from build123d import *

# Parameters (mm, degrees)
SKETCH1_W                = 9
SKETCH1_H                = 55
SKETCH1_W_2              = 91
SKETCH1_H_2              = 5
BOSS_EXTRUDE3_DEPTH      = 5
SKETCH6_W                = 18
SKETCH6_H                = 60
BOSS_EXTRUDE4_DEPTH      = 18
SKETCH7_W                = 91
SKETCH7_H                = 5
BOSS_EXTRUDE5_DEPTH      = 100
SKETCH13_W               = 18
SKETCH13_H               = 5
CUT_EXTRUDE6_DEPTH       = 75
SKETCH16_R               = 4.2
CUT_EXTRUDE7_DEPTH       = 20
CUT_EXTRUDE8_DEPTH       = 75
CUT_EXTRUDE10_DEPTH      = 8
CUT_EXTRUDE11_DEPTH      = 22
CUT_EXTRUDE14_DEPTH      = 34
CUT_EXTRUDE14_DEPTH_BACK = 5
FILLET4_R                = 10
CUT_EXTRUDE15_DEPTH      = 24
CUT_EXTRUDE15_DEPTH_BACK = 1
SKETCH23_R               = 21
SKETCH26_R               = 1.575
CUT_EXTRUDE16_DEPTH      = 10
SKETCH27_W               = 40
SKETCH27_H               = 5
BOSS_EXTRUDE6_DEPTH      = 10


with BuildPart() as part:
    # Sketch1 → Boss-Extrude3 (new body)
    with BuildSketch(Plane.XY):
        with Locations((41, -0.737170899)):
            Rectangle(SKETCH1_W, SKETCH1_H)
        with Locations((32, -0.737170899)):
            Rectangle(SKETCH1_W, SKETCH1_H)
        with BuildLine():
            Line((27.5, 26.762829101), (0, 26.762829101))
            Line((0, 26.762829101), (0, 10.812829101))
            ThreePointArc((0, 10.812829101), (8.167083323, 7.429912424), (11.55, -0.737170899))
            ThreePointArc((11.55, -0.737170899), (8.167083323, -8.904254222), (0, -12.287170899))
            Line((0, -12.287170899), (0, -28.237170899))
            Line((0, -28.237170899), (27.5, -28.237170899))
            Line((27.5, -28.237170899), (27.5, 26.762829101))
        make_face()
        with BuildLine():
            Line((0, 10.812829101), (0, 26.762829101))
            Line((0, 26.762829101), (-27.5, 26.762829101))
            Line((-27.5, 26.762829101), (-27.5, -28.237170899))
            Line((-27.5, -28.237170899), (0, -28.237170899))
            Line((0, -28.237170899), (0, -12.287170899))
            ThreePointArc((0, -12.287170899), (-11.55, -0.737170899), (0, 10.812829101))
        make_face()
        with Locations((-32, -0.737170899)):
            Rectangle(SKETCH1_W, SKETCH1_H)
        with Locations((-41, -0.737170899)):
            Rectangle(SKETCH1_W, SKETCH1_H)
        with Locations((0, 29.262829101)):
            Rectangle(SKETCH1_W_2, SKETCH1_H_2)
    extrude(amount=BOSS_EXTRUDE3_DEPTH)

    # Sketch6 → Boss-Extrude4 (add)
    with BuildSketch(Plane(origin=(0, 0, 0), x_dir=(-1, 0, 0), z_dir=(0, 0, -1))):
        with Locations((-36.5, 1.762829101)):
            Rectangle(SKETCH6_W, SKETCH6_H)
        with Locations((36.5, 1.762829101)):
            Rectangle(SKETCH6_W, SKETCH6_H)
    extrude(amount=BOSS_EXTRUDE4_DEPTH)

    # Sketch7 → Boss-Extrude5 (add)
    with BuildSketch(Plane.XY.offset(5)):
        with Locations((0, 29.262829101)):
            Rectangle(SKETCH7_W, SKETCH7_H)
    extrude(amount=BOSS_EXTRUDE5_DEPTH)

    # Sketch13 → Cut-Extrude6 (cut)
    with BuildSketch(Plane(origin=(0, 31.762829101, 0), x_dir=(1, 0, 0), z_dir=(0, 1, 0))):
        with Locations((-36.5, 15.5)):
            Rectangle(SKETCH13_W, SKETCH13_H)
        with Locations((36.5, 15.5)):
            Rectangle(SKETCH13_W, SKETCH13_H)
    extrude(amount=-CUT_EXTRUDE6_DEPTH, mode=Mode.SUBTRACT)

    # Sketch16 → Cut-Extrude7 (cut)
    with BuildSketch(Plane(origin=(0, 31.762829101, 0), x_dir=(1, 0, 0), z_dir=(0, 1, 0))):
        with Locations(Location((-36.5, 4, 0), (0, 0, 180))):
            Circle(SKETCH16_R)
        with Locations(Location((36.5, 4, 0), (0, 0, 180))):
            Circle(SKETCH16_R)
    extrude(amount=-CUT_EXTRUDE7_DEPTH, mode=Mode.SUBTRACT)

    # Sketch17 → Cut-Extrude8 (cut)
    with BuildSketch(Plane(origin=(0, 31.762829101, 0), x_dir=(1, 0, 0), z_dir=(0, 1, 0))):
        with BuildLine():
            Line((-45.5, 13), (-45.5, 4))
            ThreePointArc((-45.5, 4), (-42.863961031, 10.363961031), (-36.5, 13))
            Line((-36.5, 13), (-45.5, 13))
        make_face()
        with BuildLine():
            ThreePointArc((-36.5, 13), (-30.136038969, 10.363961031), (-27.5, 4))
            Line((-27.5, 4), (-27.5, 13))
            Line((-27.5, 13), (-36.5, 13))
        make_face()
        with BuildLine():
            Line((27.5, 13), (27.5, 4))
            ThreePointArc((27.5, 4), (30.136038969, 10.363961031), (36.5, 13))
            Line((36.5, 13), (27.5, 13))
        make_face()
        with BuildLine():
            Line((45.5, 13), (36.5, 13))
            ThreePointArc((36.5, 13), (42.863961031, 10.363961031), (45.5, 4))
            Line((45.5, 4), (45.5, 13))
        make_face()
    extrude(amount=-CUT_EXTRUDE8_DEPTH, mode=Mode.SUBTRACT)

    # Sketch18 → Cut-Extrude10 (cut)
    with BuildSketch(Plane(origin=(0, 31.762829101, 0), x_dir=(1, 0, 0), z_dir=(0, 1, 0))):
        with BuildLine():
            ThreePointArc((-45.5, -105), (-26.743051045, -83.063543967), (-20, -55))
            Line((-20, -55), (-45.5, -55))
            Line((-45.5, -55), (-45.5, -105))
        make_face()
        with BuildLine():
            Line((-45.5, -55), (-20, -55))
            ThreePointArc((-20, -55), (-26.743051045, -26.936456033), (-45.5, -5))
            Line((-45.5, -5), (-45.5, -55))
        make_face()
        with BuildLine():
            ThreePointArc((-45.5, -105), (-26.743051045, -83.063543967), (-20, -55))
            Line((-20, -55), (-45.5, -55))
            Line((-45.5, -55), (-45.5, -105))
        make_face()
        with BuildLine():
            Line((-45.5, -55), (-20, -55))
            ThreePointArc((-20, -55), (-26.743051045, -26.936456033), (-45.5, -5))
            Line((-45.5, -5), (-45.5, -55))
        make_face()
        with BuildLine():
            Line((-20, -105), (-20, -55))
            ThreePointArc((-20, -55), (-26.743051045, -83.063543967), (-45.5, -105))
            Line((-45.5, -105), (-20, -105))
        make_face()
        with BuildLine():
            Line((20, -55), (20, -105))
            Line((20, -105), (45.5, -105))
            ThreePointArc((45.5, -105), (26.743051045, -83.063543967), (20, -55))
        make_face()
        with BuildLine():
            Line((45.5, -55), (45.5, -5))
            ThreePointArc((45.5, -5), (26.743051045, -26.936456033), (20, -55))
            Line((20, -55), (45.5, -55))
        make_face()
        with BuildLine():
            ThreePointArc((20, -55), (26.743051045, -83.063543967), (45.5, -105))
            Line((45.5, -105), (45.5, -55))
            Line((45.5, -55), (20, -55))
        make_face()
        with BuildLine():
            Line((45.5, -55), (45.5, -5))
            ThreePointArc((45.5, -5), (26.743051045, -26.936456033), (20, -55))
            Line((20, -55), (45.5, -55))
        make_face()
        with BuildLine():
            ThreePointArc((20, -55), (26.743051045, -83.063543967), (45.5, -105))
            Line((45.5, -105), (45.5, -55))
            Line((45.5, -55), (20, -55))
        make_face()
    extrude(amount=-CUT_EXTRUDE10_DEPTH, mode=Mode.SUBTRACT)

    # Sketch19 → Cut-Extrude11 (cut)
    with BuildSketch(Plane.XY.offset(5)):
        with BuildLine():
            Line((-32.5, -0.737170899), (-45.5, -0.737170899))
            Line((-45.5, -0.737170899), (-45.5, -28.237170899))
            Line((-45.5, -28.237170899), (-17.320508076, -28.237170899))
            ThreePointArc((-17.320508076, -28.237170899), (-28.453176558, -16.442798673), (-32.5, -0.737170899))
        make_face()
        with BuildLine():
            Line((45.5, -28.237170899), (17.320508076, -28.237170899))
            ThreePointArc((17.320508076, -28.237170899), (28.453176558, -16.442798673), (32.5, -0.737170899))
            Line((32.5, -0.737170899), (45.5, -0.737170899))
            Line((45.5, -0.737170899), (45.5, -28.237170899))
        make_face()
    extrude(amount=-CUT_EXTRUDE11_DEPTH, mode=Mode.SUBTRACT)

    # Sketch21 → Cut-Extrude14 (cut, two sides: drawn at the far end of the back side and taken through both)
    with BuildSketch(Plane.XZ.offset(0.737170899).offset(-CUT_EXTRUDE14_DEPTH_BACK)):
        with BuildLine():
            Line((27.5, 0), (32.5, 0))
            Line((32.5, 0), (32.5, 5))
            Line((32.5, 5), (45.5, 5))
            Line((45.5, 5), (45.5, -4))
            ThreePointArc((45.5, -4), (36.5, -13), (27.5, -4))
            Line((27.5, -4), (27.5, 0))
        make_face()
        with BuildLine():
            Line((-27.5, -4), (-27.5, 0))
            Line((-27.5, 0), (-32.5, 0))
            Line((-32.5, 0), (-32.5, 5))
            Line((-32.5, 5), (-45.5, 5))
            Line((-45.5, 5), (-45.5, -4))
            ThreePointArc((-45.5, -4), (-36.5, -13), (-27.5, -4))
        make_face()
    extrude(amount=CUT_EXTRUDE14_DEPTH + CUT_EXTRUDE14_DEPTH_BACK, mode=Mode.SUBTRACT)

    # Fillet4
    # the kernel refuses this fillet: 10 mm, written as the material it adds along each edge
    with BuildSketch(Plane(origin=(70.5, 26.762829101, 5), x_dir=(0, -1, 0), z_dir=(-1, 0, 0))) as fillet4_piece_1_section:
        with BuildLine():
            CenterArc((FILLET4_R, FILLET4_R), FILLET4_R, 180, 90)
            Line((0, FILLET4_R), (0, 0))
            Line((0, 0), (FILLET4_R, 0))
        make_face()
    fillet4_piece_1 = extrude(amount=141, mode=Mode.PRIVATE)
    fillet4_piece_1 = fillet4_piece_1 - Plane(origin=(-81.769607843, 24.471447362, 55), x_dir=(0.5871756209824568, 0, 0.8094595667010591), z_dir=(0, 1, 0)) * Cylinder(61.769607843, 322, mode=Mode.PRIVATE)
    fillet4_piece_1 = fillet4_piece_1 - Plane(origin=(81.769607843, 24.471447362, 55), x_dir=(-0.5871756209824566, 0, -0.8094595667010592), z_dir=(0, 1, 0)) * Cylinder(61.769607843, 322, mode=Mode.PRIVATE)
    add(fillet4_piece_1)

    # Sketch23 → Cut-Extrude15 (cut, two sides: drawn at the far end of the back side and taken through both)
    with BuildSketch(Plane.XY.offset(5).offset(-CUT_EXTRUDE15_DEPTH_BACK)):
        with Locations(Location((0, -0.737170899, 0), (0, 0, 123.557309762))):
            Circle(SKETCH23_R)
    extrude(amount=CUT_EXTRUDE15_DEPTH + CUT_EXTRUDE15_DEPTH_BACK, mode=Mode.SUBTRACT)

    # Sketch26 → Cut-Extrude16 (cut)
    with BuildSketch(Plane.XY.offset(4)):
        with Locations((0, -16.487170899)):
            Circle(SKETCH26_R)
        with Locations((-13.63990011, 7.137829101)):
            Circle(SKETCH26_R)
        with Locations((13.63990011, 7.137829101)):
            Circle(SKETCH26_R)
    extrude(amount=-CUT_EXTRUDE16_DEPTH, mode=Mode.SUBTRACT)

    # Sketch27 → Boss-Extrude6 (add)
    with BuildSketch(Plane.XY.offset(105)):
        with Locations((0, 29.262829101)):
            Rectangle(SKETCH27_W, SKETCH27_H)
    extrude(amount=BOSS_EXTRUDE6_DEPTH)


solid = part.part
Work out the finished part from the listing and answer in its coordinate system (mm). A direction names the side the tool comes from. Give positions to 0.01 mm unless a question says otherwise; leave off trailing zeros. Loops run counter-clockwise (first coordinate to the right, second up) from the corner with the lowest first, then second, coordinate; pieces in that order, holes last. Notation, with made-up numbers: (20, 17.25) - (45, 17.25) arc R16 cw to (45, 33.25) - close; hole circle Ø11 at (59.25, 0). An arc over 180 degrees is marked (long way). Answer in a Markdown table with one row per item.
(1) Consider L1, parallel to Y at x = 0, z = 0.85; L2, parallel to Y at x = 14.5, z = 76; L3, parallel to X at y = 15, z = -2. Determine where each line is inside the solid, lowest interval first. Write a range as [from, to].
Results list:
| item | result |
|---|---|
| L1 | y = [-28.24, -18.06], [-14.91, -12.29], [10.81, 31.76] |
| L2 | y = [26.76, 31.76] |
| L3 | x = [-45.5, -40.19], [-32.81, -27.5], [27.5, 32.81], [40.19, 45.5] |
(2) Flat-ended cylindrical pins translate along their axes: pin 1 Ø5.5 at (y, z) = (2, 1.5) entering from +X; pin 2 Ø8 at (x, y) = (-13.5, 11.5) entering from +Z; pin 3 Ø18 at (x, y) = (3.5, 13.5) entering from -Z; pin 4 Ø5 at (x, y) = (-13.64, 7.14) entering from +Z. Find the tip coordinate at first contact, or state that the pin passes through.
Results list:
| item | result |
|---|---|
| pin 1 | stops at x = 45.5 |
| pin 2 | stops at z = 5 |
| pin 3 | stops at z = 0 |
| pin 4 | stops at z = 4 |
(3) For a pull along Y with two mould halves and no side action, classify faces 1 (the face through (-27.5, 18, -2)), 2 (the face through (0.637, 23.911, 8.007)), 3 (the face through (12.39, 6.18, 2.03)), 4 (the face through (-1, 31.763, 50)) as pulls with the +Y half, pulls with the -Y half, needs draft (parallel to the pull), parting line crosses it, or undercut.
Results list:
| item | result |
|---|---|
| face 1 | needs draft |
| face 2 | pulls with the -Y half |
| face 3 | undercut |
| face 4 | pulls with the +Y half |
(4) Section C-C (z = 24) is taken. Give the vertices of the cut face in (x, y).
Results list:
| item | result |
|---|---|
| outline | (-28.34, 26.76) - (28.34, 26.76) - (28.34, 31.76) - (-28.34, 31.76) - close |
(5) Section A-A (y = 24) is taken. Give the vertices of the cut face in (x, z).
Results list:
| item | result |
|---|---|
| outline | (-45.5, -4) arc R9 ccw to (-27.5, -4) - (-27.5, 0) - (27.5, 0) - (27.5, -4) arc R9 ccw to (45.5, -4) - (45.5, 5) arc R61.77 cw to (41.57, 8.1) - (-41.57, 8.1) arc R61.77 cw to (-45.5, 5) - close; hole circle Ø8.4 at (-36.5, -4); hole circle Ø8.4 at (36.5, -4) |
(6) A tool of negligible diameter and unlimited length cuts with its end or side. For faces 5 (the face through (-20, 29, 85)), 6 (the face through (-32.5, 2, 2)), 7 (the face through (20, 29, 85)), 8 (the face through (32.494, 21.903, -2.738)), from which of +Z, -Z, +X, -X, +Y, -Y can it reach the whole face along a straight path? Write none if from no direction.
Results list:
| item | result |
|---|---|
| face 5 | +Z, -X, +Y, -Y |
| face 6 | +Z, -Z, -X, -Y |
| face 7 | +Z, +X, +Y, -Y |
| face 8 | +Y |
(7) Section B-B (z = 100.5) is taken. Give the vertices of the cut face in (x, y).
Results list:
| item | result |
|---|---|
| outline | (-20, 26.76) - (20, 26.76) - (20, 31.76) - (-20, 31.76) - close |
